Here's the drawing with two shaded views (mm, measured from the low corner). I have some questions. Round coordinates to 2 decimals unless told otherwise and drop trailing zeros. Order: outer loops, then holes, each group sorted by start corner. A loop starts at its lowest first (then second) coordinate and runs counter-clockwise, first axis right, second up.
Q1. If we section it at C-C (z = 2.5): Please give me the cut outline in (x, y), plus the area to 3 significant figures.
Q2. If we section it at A-A (x = 20): Please give me the cut outline in (y, z), plus the area to 3 significant figures.
Q3. We'd pull the mould along Y, two halves only. Please class the marked faces 1, 2, 3 and 4: pulls with the +Y half, pulls with the -Y half, needs draft (parallel to the pull), parting line crosses it, or undercut.
Q4. If we section it at B-B (z = 28.5): Please give me the cut outline in (x, y).
Q5. If I drill on line 1 (Y direction, x = 24.5, z = 2); line 2 (Y direction, x = 20, z = 6.5); line 3 (Z direction, x = 17.5, y = 24.5), over which ranges is the centre line in solid material (lowest first)?
Q6. Will these pins go through, and if not, where does the flat tip stop? P1, Ø6, axis at x = 11, z = 6, coming from the -Y side; P2, Ø2, axis at y = 15, z = 20, coming from the +X side; P3, Ø12, axis at y = 25, z = 12, coming from the +X side.
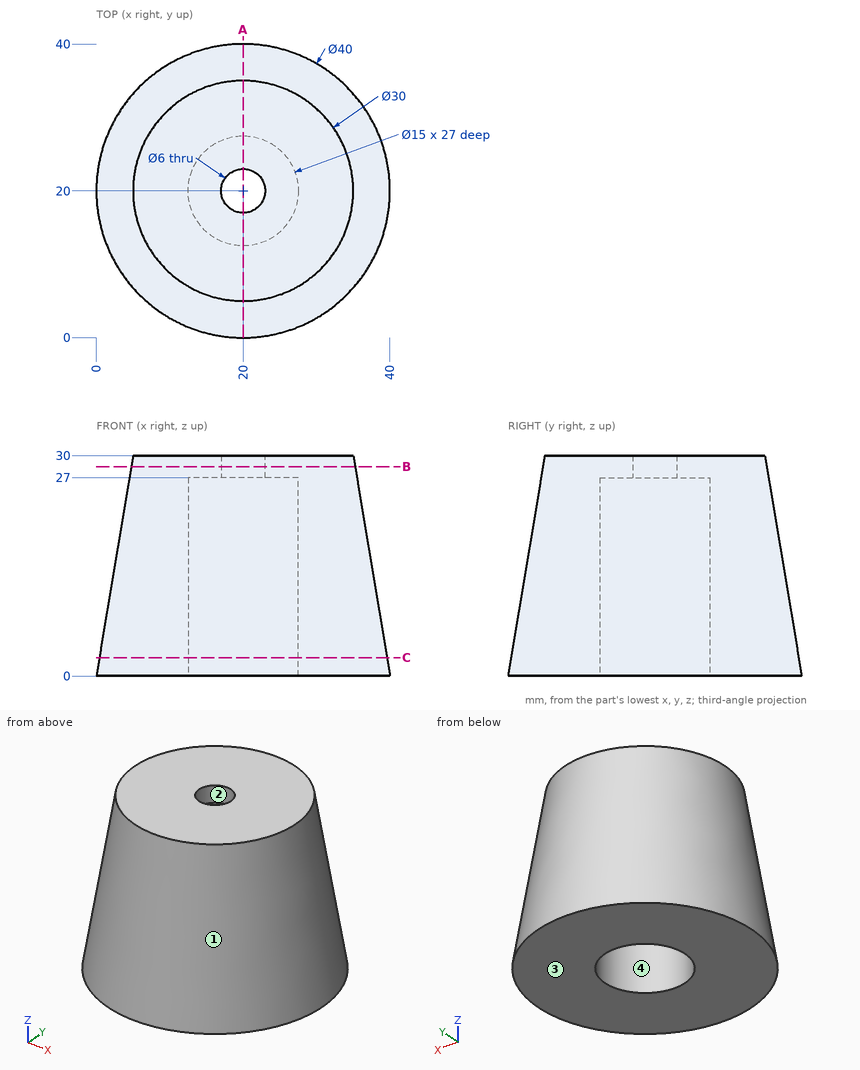
Solution:
1. outline: circle Ø39.17 at (20, 20); hole circle Ø15 at (20, 20)
1. area: 1,030 mm2
2. outline: (0, 0) - (12.5, 0) - (12.5, 27) - (17, 27) - (17, 30) - (5, 30) - close; (23, 27) - (27.5, 27) - (27.5, 0) - (40, 0) - (35, 30) - (23, 30) - close
2. area: 627 mm2
3. face 1: parting line crosses it
3. face 2: undercut
3. face 3: needs draft
3. face 4: undercut
4. outline: circle Ø30.5 at (20, 20); hole circle Ø6 at (20, 20)
5. line 1: y = 0.86 to 14, 26 to 39.14
5. line 2: y = 1.08 to 12.5, 27.5 to 38.92
5. line 3: z = 27 to 30
6. P1: stops at y = 1.84
6. P2: stops at x = 36.23
6. P3: stops at x = 38.76
